Design review of the part built by this model. Coordinates are the model's own, in mm. A direction names the side the tool comes from. Coordinates: 2 decimals unless noted, no trailing zeros. Loops run counter-clockwise (first coordinate to the right, second up) from the corner with the lowest first, then second, coordinate; pieces in that order, holes last. Notation, with made-up numbers: M 24.5,19 L 38.5,19 A18 cw 38.5,27 Z; hole C -28,-18.75 d2. An arc over 180 degrees is marked long. Answer as CSV lines item,"result". Start each with the question number.
from build123d import *

# Parameters (mm, degrees)
F0_W     = 4
F0_H     = 543
F1_DEPTH = 800
F2_W     = 6
F2_H     = 543
F3_DEPTH = 4


with BuildPart() as f1:
    # F0 (on Front) → F1 (new body)
    with BuildSketch(Plane.XZ):
        with Locations((2, 271.5)):
            Rectangle(F0_W, F0_H)
        Polygon((4, 0), (0, 0), (73.972428, -75.628935), (76.831998, -72.831998), align=None)
    extrude(amount=F1_DEPTH)

    # F2 (on face) → F3 (join)
    with BuildSketch(Plane.YZ.offset(4)):
        with Locations((-803, 271.5)):
            Rectangle(F2_W, F2_H)
        with Locations((3, 271.5)):
            Rectangle(F2_W, F2_H)
    extrude(amount=-F3_DEPTH)


solid = f1.part
Item 1: Add section A-A (y = -496). Give the boundary of the cut face in (x, z).
Item 2: For line 1 along X through (y, z) = (-223.5, 356.5); line 2 along Z through (x, y) = (69, -528.5); line 3 along Z through (x, y) = (45, -524), list the stretches that pass through material, from the lowest coordinate up. Write a range as from..to.
Item 3: For faces 1 (the face through (36.468, -394.4, -37.285)), 2 (the face through (4, -406, 275)), list the 3-axis set-ups (+Z, -Z, +X, -X, +Y, -Y) from which the entire face can be reached by the end or side of a thin tool; tool diameter is ignored.
Item 4: For pin 1 (4.5 mm diameter, centred on x = 3, y = -802, fed in from -Z); pin 2 (2 mm diameter, centred on x = 3, y = 4, fed in from -Z); pin 3 (1.5 mm diameter, centred on y = -627.5, z = 37.5, fed in from +X), all flat-tipped, find the tip position at first contact; note any pin that passes through.
Item 5: Add section B-B (z = 356.5). Give the boundary of the cut face in (x, y), plus the area to 3 significant figures.
Item 6: Add section C-C (x = 27.5). Give the boundary of the cut face in (y, z).
Response:
1,outline,"M 0,0 L 73.97,-75.63 L 76.83,-72.83 L 4,0 L 4,543 L 0,543 Z"
2,line 1,"0..4"
2,line 2,"-70.55..-65"
2,line 3,"-46.01..-41"
3,face 1,"-Z, -X, +Y, -Y"
3,face 2,"+Z, +X, +Y, -Y"
4,pin 1,"z = -4.12"
4,pin 2,"z = 0"
4,pin 3,"x = 4"
5,outline,"M 0,-806 L 4,-806 L 4,6 L 0,6 Z"
5,area,"3,250 mm²"
6,outline,"M -800,-28.12 L 0,-28.12 L 0,-23.5 L -800,-23.5 Z"
